from build123d import *

# Parameters (mm, degrees)
SKETCH1_R           = 1.5
BOSS_EXTRUDE1_DEPTH = 2


with BuildPart() as part:
    # Sketch1 → Boss-Extrude1 (new body)
    with BuildSketch(Plane.XY):
        with BuildLine():
            Line((10, -1.562186701), (8, -1.562186701))
            Line((8, -1.562186701), (8, -3.062186701))
            Line((8, -3.062186701), (4, -3.062186701))
            Line((4, -3.062186701), (4, -7.937813299))
            Line((4, -7.937813299), (-10, -7.937813299))
            Line((-10, -7.937813299), (-10, 2.937813299))
            ThreePointArc((-10, 2.937813299), (-8.535533906, 6.473347205), (-5, 7.937813299))
            Line((-5, 7.937813299), (8, 7.937813299))
            Line((8, 7.937813299), (8, 6.437813299))
            Line((8, 6.437813299), (10, 6.437813299))
            Line((10, 6.437813299), (10, -1.562186701))
        make_face()
        with Locations((-6.439339828, 4.377153127)):
            Circle(SKETCH1_R, mode=Mode.SUBTRACT)
    extrude(amount=BOSS_EXTRUDE1_DEPTH)


solid = part.part
Geometry: final body of the model. Coordinates: model frame, mm. A direction names the side the tool comes from. Coordinates: 2 decimals unless noted, no trailing zeros. Write each loop counter-clockwise with the first axis right and the second up, starting at its lowest first coordinate (ties: lowest second). Pieces come first, ordered by that corner, then holes. Notation, with made-up numbers: (-2, 13) - (26, 13) arc R22 ccw to (26, 29) - close; hole circle Ø1 at (73.25, 84.5). An arc over 180 degrees is marked (long way). Return JSON: item names as keys, results as strings.
Item 1: Section query B-B (z = 1.1). Output: boundary loops of the cut face in (x, y).
Completed:
{"outline": "(-10, -7.94) - (4, -7.94) - (4, -3.06) - (8, -3.06) - (8, -1.56) - (10, -1.56) - (10, 6.44) - (8, 6.44) - (8, 7.94) - (-5, 7.94) arc R5 ccw to (-10, 2.94) - close; hole circle Ø3 at (-6.44, 4.38)"}
Item 2: Section query A-A (x = -5.5). Output: boundary loops of the cut face in (y, z).
Completed:
{"outline": "(-7.94, 0) - (3.21, 0) - (3.21, 2) - (-7.94, 2) - close; (5.55, 0) - (7.91, 0) - (7.91, 2) - (5.55, 2) - close"}
Item 3: Pin query (flat end, axial travel): pin 1 Ø1 at (x, z) = (5, 1.5) entering from -Y; pin 2 Ø1 at (x, z) = (9, 1) entering from -Y; pin 3 Ø0.8 at (y, z) = (-2.5, 0.5) entering from +X. Return the tip coordinate at first contact, or that it passes through.
Completed:
{"pin 1": "stops at y = -3.06", "pin 2": "stops at y = -1.56", "pin 3": "stops at x = 8"}
Item 4: Section query C-C (x = 7). Output: boundary loops of the cut face in (y, z).
Completed:
{"outline": "(-3.06, 0) - (7.94, 0) - (7.94, 2) - (-3.06, 2) - close"}
Item 5: Line query: L1, parallel to Y at x = 7.25, z = 1.15; L2, parallel to X at y = -6.5, z = 0.2; L3, parallel to Y at x = -6, z = 0.35. Output: solid intervals per line, ascending.
Completed:
{"L1": "y = -3.06 to 7.94", "L2": "x = -10 to 4", "L3": "y = -7.94 to 2.94, 5.81 to 7.84"}
Item 6: Reachability of faces 1 (the face through (8, 7, 1)), 2 (the face through (6, -3.062, 1)), 3 (the face through (-8.574, 6.434, 0.986)) from +Z, -Z, +X, -X, +Y, -Y: full face, straight path, thin tool, end or side. Return the list, or none.
Completed:
{"face 1": "+Z, -Z, +X, +Y", "face 2": "+Z, -Z, +X, -Y", "face 3": "+Z, -Z, -X, +Y"}
Item 7: Pull-direction query (Y, two-part tool) for faces 4 (the face through (1, 7.938, 1)), 5 (the face through (8, -2, 1)), 6 (the face through (-5.054, 3.803, 0.986)), 7 (the face through (9, -1.562, 1)); classes: +Y half, -Y half, draft (parallel to the pull), parting line (faces both ways), or undercut.
Completed:
{"face 4": "+Y half", "face 5": "draft", "face 6": "undercut", "face 7": "-Y half"}
